```python
from build123d import *

# Parameters (mm, degrees)
F0_R        = 50.8
F1_DEPTH    = 6.35
F2_R        = 3.3872020891
F3_DEPTH    = 50.8
F4_W        = 3.7956816162
F4_H        = 11.7751168936
F4_W_2      = 3.9597040755
F4_H_2      = 12.2920670431
F4_W_3      = 3.7532411516
F4_H_3      = 11.5020200028
F4_W_4      = 4.1028857231
F4_H_4      = 11.3390376209
F5_DEPTH    = 17.78
F6_R        = 5.08
F7_DEPTH    = 25.4
F8_T1_DEPTH = 36.0204370388
F8_T3_DEPTH = 36.2647510961
F8_T5_DEPTH = 36.3499649547
F8_T7_DEPTH = 37.0667199375
F9_R        = 2.6244366773
F9_R_2      = 2.7684987857
F9_R_3      = 3.2478511369
F10_DEPTH   = 25.4


# Not quite as in the source:
# - a fillet or chamfer that OpenCascade refuses, or shapes differently, is made with other operations: its cross-section is extruded or revolved along the edge and cut away or added


with BuildPart() as f1:
    # F0 (on Top) → F1 (new body)
    with BuildSketch(Plane.XY):
        Circle(F0_R)
    extrude(amount=F1_DEPTH)

    # F2 (on Top) → F3 (join)
    with BuildSketch(Plane.XY):
        Circle(F2_R)
    extrude(amount=F3_DEPTH)

    # F4 (on face) → F5 (join)
    with BuildSketch(Plane.XY.offset(6.35)):
        with Locations((22.9978772923, 5.7736401254)):
            Rectangle(F4_W, F4_H)
        with Locations((44.0967701382, 5.7131922383)):
            Rectangle(F4_W_2, F4_H_2)
        with Locations((-42.1600081027, 5.5507384532)):
            Rectangle(F4_W_3, F4_H_3)
        with Locations((-24.7639858169, 5.4692472622)):
            Rectangle(F4_W_4, F4_H_4)
    extrude(amount=F5_DEPTH)

    # F6
    f6_edges = [f1.edges().sort_by_distance(p)[0] for p in [
        (24.895718, 5.77364, 6.35),
        (42.116918, 5.713192, 6.35),
        (-40.283388, 5.550738, 6.35),
        (-26.815429, 5.469247, 6.35),
    ]]
    fillet(f6_edges, radius=F6_R)

    # F4 (on face) → F7 (join)
    with BuildSketch(Plane.XY.offset(6.35)):
        with Locations((22.9978772923, 5.7736401254)):
            Rectangle(F4_W, F4_H)
        with Locations((44.0967701382, 5.7131922383)):
            Rectangle(F4_W_2, F4_H_2)
        with Locations((-42.1600081027, 5.5507384532)):
            Rectangle(F4_W_3, F4_H_3)
        with Locations((-24.7639858169, 5.4692472622)):
            Rectangle(F4_W_4, F4_H_4)
    extrude(amount=F7_DEPTH)

    # F8: fillet of radius 5.08 on 4 edges, made by hand

    # F8_s2 → F8_t1 (cut)
    with BuildSketch(Plane.XZ.offset(-23.5609569726)):
        with BuildLine():
            ThreePointArc((-40.2833875269, 31.75), (-42.9906301007, 29.9339099153), (-44.0366286784, 26.8463165928))
            Line((-44.0366286784, 26.8463165928), (-44.0366286784, 31.75))
            Line((-44.0366286784, 31.75), (-40.2833875269, 31.75))
        make_face()
    extrude(amount=F8_T1_DEPTH, mode=Mode.SUBTRACT)

    # F8_s4 → F8_t3 (cut)
    with BuildSketch(Plane.XZ.offset(-23.6016228103)):
        with BuildLine():
            ThreePointArc((-26.8154286784, 31.75), (-23.8701622671, 29.9930657457), (-22.7125429553, 26.764857305))
            Line((-22.7125429553, 26.764857305), (-22.7125429553, 31.75))
            Line((-22.7125429553, 31.75), (-26.8154286784, 31.75))
        make_face()
    extrude(amount=F8_T3_DEPTH, mode=Mode.SUBTRACT)

    # F8_s6 → F8_t5 (cut)
    with BuildSketch(Plane.XZ.offset(-23.9486226027)):
        with BuildLine():
            ThreePointArc((24.8957181004, 31.75), (22.1594185349, 29.9400314031), (21.1000364843, 26.8350303878))
            Line((21.1000364843, 26.8350303878), (21.1000364843, 31.75))
            Line((21.1000364843, 31.75), (24.8957181004, 31.75))
        make_face()
    extrude(amount=F8_T5_DEPTH, mode=Mode.SUBTRACT)

    # F8_s8 → F8_t7 (cut)
    with BuildSketch(Plane.XZ.offset(-24.2465522071)):
        with BuildLine():
            ThreePointArc((42.1169181004, 31.75), (44.9650918619, 29.9664489871), (46.0766221759, 26.7950694211))
            Line((46.0766221759, 26.7950694211), (46.0766221759, 31.75))
            Line((46.0766221759, 31.75), (42.1169181004, 31.75))
        make_face()
    extrude(amount=F8_T7_DEPTH, mode=Mode.SUBTRACT)

    # F9 (on face) → F10 (cut)
    with BuildSketch(Plane.XY.offset(6.35)):
        with Locations((0, 43.9927652478)):
            Circle(F9_R)
        with Locations((34.4810411334, 29.0996860713)):
            Circle(F9_R_2)
        with Locations((-36.2776443362, 28.5628065467)):
            Circle(F9_R_3)
    extrude(amount=-F10_DEPTH, mode=Mode.SUBTRACT)


solid = f1.part
```
Source: CAD feature listing. Evaluate the final solid. Frame: model axes, mm. A direction names the side the tool comes from. Give positions to 0.01 mm unless a question says otherwise; leave off trailing zeros. Order: outer loops, then holes, each group sorted by start corner. A loop starts at its lowest first (then second) coordinate and runs counter-clockwise, first axis right, second up.
(1) Access query for faces 5 (the face through (-25, -0.2, 19)), 6 (the face through (44, 11.859, 19)), 7 (the face through (40.59, 5.8, 7.8)), 8 (the face through (46.077, 6, 16)). Directions: +Z, -Z, +X, -X, +Y, -Y. A direction counts if a zero-diameter tool reaches every point of the face in a straight line with its end or side. Return the directions, or none.
(2) Contact query for flat-ended pins moving along their axis: P1, Ø3.5, axis at y = 2.5, z = 14.5, coming from the -X side; P2, Ø10, axis at x = -19, y = -12.5, coming from the +Z side; P3, Ø3.5, axis at y = 7, z = 22, coming from the +X side. Output: stop coordinate, or through.
(3) Section query A-A (x = 0). Return the cut outline in (y, z), plus the area to 3 significant figures.
(4) Material intervals for line 1 along X through (y, z) = (31.5, 5); line 2 along X through (y, z) = (2, 8.5); line 3 along Y through (x, z) = (0, 3), sorted ascending.
(5) Section query B-B (z = 13). Return the cut outline in (x, y), plus the area to 3 significant figures.
(6) Section query C-C (z = 29). Return the cut outline in (x, y).
(7) Section query D-D (y = 1.5). Return the cut outline in (x, z).
(8) Pull-direction query (Y, two-part tool) for faces 1 (the face through (-42, -0.2, 19)), 2 (the face through (-40.283, 5, 21)), 3 (the face through (-38.86, 26.59, 3.22)), 4 (the face through (-0.3, 46.6, 3.2)); classes: +Y half, -Y half, draft (parallel to the pull), parting line (faces both ways), or undercut.
Outcome:
1. face 5: +Z, -X, -Y
1. face 6: +Z, +X, -X, +Y
1. face 7: +Z, +Y, -Y
1. face 8: +Z, +X, +Y, -Y
2. P1: stops at x = -44.04
2. P2: stops at z = 6.35
2. P3: stops at x = 46.08
3. outline: (-50.8, 0) - (41.37, 0) - (41.37, 6.35) - (3.39, 6.35) - (3.39, 50.8) - (-3.39, 50.8) - (-3.39, 6.35) - (-50.8, 6.35) - close; (46.62, 0) - (50.8, 0) - (50.8, 6.35) - (46.62, 6.35) - close
3. area: 913 mm2
4. line 1: x = -39.85 to -37.66, -34.89 to 33.1, 35.86 to 39.85
4. line 2: x = -44.04 to -39.35, -27.75 to -22.71, -2.73 to 2.73, 21.1 to 25.83, 41.19 to 46.08
4. line 3: y = -50.8 to 41.37, 46.62 to 50.8
5. outline: (-44.04, -0.2) - (-40.28, -0.2) - (-40.28, 11.3) - (-44.04, 11.3) - close; (-26.82, -0.2) - (-22.71, -0.2) - (-22.71, 11.14) - (-26.82, 11.14) - close; circle Ø6.77 at (0, 0); (21.1, -0.11) - (24.9, -0.11) - (24.9, 11.66) - (21.1, 11.66) - close; (42.12, -0.43) - (46.08, -0.43) - (46.08, 11.86) - (42.12, 11.86) - close
5. area: 219 mm2
6. outline: (-43.56, -0.2) - (-40.28, -0.2) - (-40.28, 11.3) - (-43.56, 11.3) - close; (-26.82, -0.2) - (-23.23, -0.2) - (-23.23, 11.14) - (-26.82, 11.14) - close; circle Ø6.77 at (0, 0); (21.58, -0.11) - (24.9, -0.11) - (24.9, 11.66) - (21.58, 11.66) - close; (42.12, -0.43) - (45.57, -0.43) - (45.57, 11.86) - (42.12, 11.86) - close
7. outline: (-50.78, 0) - (50.78, 0) - (50.78, 6.35) - (46.08, 6.35) - (46.08, 26.8) arc R5.08 ccw to (42.12, 31.75) - (42.12, 11.43) arc R5.08 cw to (37.04, 6.35) - (29.98, 6.35) arc R5.08 cw to (24.9, 11.43) - (24.9, 31.75) arc R5.08 ccw to (21.1, 26.84) - (21.1, 6.35) - (3.04, 6.35) - (3.04, 50.8) - (-3.04, 50.8) - (-3.04, 6.35) - (-22.71, 6.35) - (-22.71, 26.76) arc R5.08 ccw to (-26.82, 31.75) - (-26.82, 11.43) arc R5.08 cw to (-31.9, 6.35) - (-35.2, 6.35) arc R5.08 cw to (-40.28, 11.43) - (-40.28, 31.75) arc R5.08 ccw to (-44.04, 26.85) - (-44.04, 6.35) - (-50.78, 6.35) - close
8. face 1: -Y half
8. face 2: draft
8. face 3: undercut
8. face 4: undercut
